Read the model definition and answer for the solid it produces. Units are mm, in the model's axes. Give positions to 0.01 mm unless a question says otherwise; leave off trailing zeros. Loops run counter-clockwise (first coordinate to the right, second up) from the corner with the lowest first, then second, coordinate; pieces in that order, holes last.
(1) Straight lines are drawn through the part: probe 1 along Z at (x, y) = (7.5, 479); probe 2 along X at (y, z) = (317.5, 20.05); probe 3 along X at (y, z) = (562, -23). For each, find the intervals that lie inside material, in ascending order.
(2) Find section B-B, the plane z = -14. Write down the section's boundary in (x, y).
(3) Find section A-A, the plane y = 378.5. Write down the section's boundary in (x, z).
(4) Each of these flat-tipped pins is pushed along its axis until it touches: P1, Ø4, axis at y = 452, z = -11, coming from the +X side; P2, Ø4, axis at x = 8, y = 305.5, coming from the -Z side; P3, Ø12, axis at x = -9, y = 530.5, coming from the -Z side. Where does it stop, or does it pass through?
```python
from build123d import *

# Parameters (mm, degrees)
F1_DEPTH = 609.6
F2_R     = 3.175
F3_DEPTH = 25.4
F4_R     = 2.54


with BuildPart() as f1:
    # F0 (on Front) → F1 (new body)
    with BuildSketch(Plane.XZ):
        with BuildLine():
            Line((-16.424578, 19.260229), (12.06593, 19.260229))
            Line((12.06593, 19.260229), (12.06593, 20.758829))
            Line((12.06593, 20.758829), (-16.653178, 20.758829))
            ThreePointArc((-16.653178, 20.758829), (-22.041332, 18.526982), (-24.273178, 13.138829))
            Line((-24.273178, 13.138829), (-24.273178, -23.307944))
            ThreePointArc((-24.273178, -23.307944), (-21.449279, -26.988121), (-17.163621, -25.212944))
            Line((-17.163621, -25.212944), (-4.463621, -3.215899))
            Line((-4.463621, -3.215899), (-5.761447, -2.466599))
            Line((-5.761447, -2.466599), (-18.034874, -23.724797))
            ThreePointArc((-18.034874, -23.724797), (-20.891979, -24.908249), (-22.774578, -22.454797))
            Line((-22.774578, -22.454797), (-22.774578, 12.910229))
            ThreePointArc((-22.774578, 12.910229), (-20.914706, 17.400357), (-16.424578, 19.260229))
        make_face()
    extrude(amount=-F1_DEPTH)

    # F2 (on face) → F3 (cut)
    with BuildSketch(Plane.XY.offset(20.758829)):
        with Locations((-0.63407, 12.7)):
            Circle(F2_R)
        with Locations((-0.63407, 38.1)):
            Circle(F2_R)
        with Locations((-0.63407, 63.5)):
            Circle(F2_R)
        with Locations((-0.63407, 88.9)):
            Circle(F2_R)
        with Locations((-0.63407, 114.3)):
            Circle(F2_R)
        with Locations((-0.63407, 139.7)):
            Circle(F2_R)
        with Locations((-0.63407, 165.1)):
            Circle(F2_R)
        with Locations((-0.63407, 190.5)):
            Circle(F2_R)
        with Locations((-0.63407, 215.9)):
            Circle(F2_R)
        with Locations((-0.63407, 241.3)):
            Circle(F2_R)
        with Locations((-0.63407, 266.7)):
            Circle(F2_R)
        with Locations((-0.63407, 292.1)):
            Circle(F2_R)
        with Locations((-0.63407, 317.5)):
            Circle(F2_R)
        with Locations((-0.63407, 342.9)):
            Circle(F2_R)
        with Locations((-0.63407, 368.3)):
            Circle(F2_R)
        with Locations((-0.63407, 393.7)):
            Circle(F2_R)
        with Locations((-0.63407, 419.1)):
            Circle(F2_R)
        with Locations((-0.63407, 444.5)):
            Circle(F2_R)
        with Locations((-0.63407, 469.9)):
            Circle(F2_R)
        with Locations((-0.63407, 495.3)):
            Circle(F2_R)
        with Locations((-0.63407, 520.7)):
            Circle(F2_R)
        with Locations((-0.63407, 546.1)):
            Circle(F2_R)
        with Locations((-0.63407, 571.5)):
            Circle(F2_R)
        with Locations((-0.63407, 596.9)):
            Circle(F2_R)
    extrude(amount=-F3_DEPTH, mode=Mode.SUBTRACT)

    # F4
    f4_edges = [f1.edges().sort_by_distance(p)[0] for p in [
        (12.06593, 0, 20.009529),
        (-5.112534, 0, -2.841249),
        (-5.112534, 609.6, -2.841249),
        (12.06593, 609.6, 20.009529),
    ]]
    fillet(f4_edges, radius=F4_R)


solid = f1.part
```
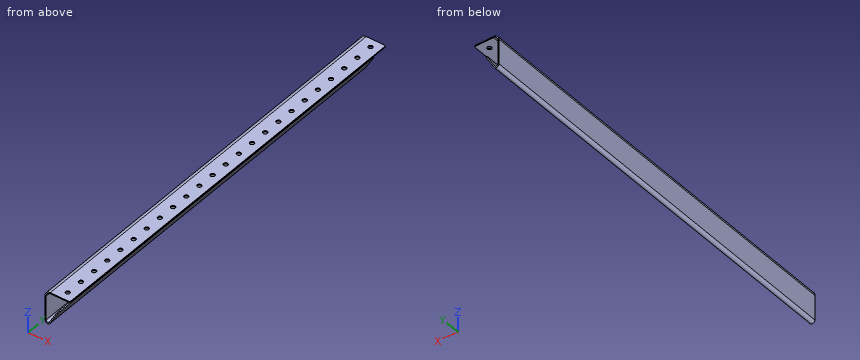
Entries:
1. probe 1: z = 19.26 to 20.76
1. probe 2: x = -19.86 to -3.81, 2.54 to 12.07
1. probe 3: x = -24.27 to -22.72, -17.62 to -15.89
2. outline: (-24.27, 0) - (-22.77, 0) - (-22.77, 609.6) - (-24.27, 609.6) - close; (-12.42, 0) - (-10.69, 0) - (-10.69, 609.6) - (-12.42, 609.6) - close
3. outline: (-24.27, -23.31) arc R3.81 ccw to (-17.16, -25.21) - (-4.46, -3.22) - (-5.76, -2.47) - (-18.03, -23.72) arc R2.54 cw to (-22.77, -22.45) - (-22.77, 12.91) arc R6.35 cw to (-16.42, 19.26) - (12.07, 19.26) - (12.07, 20.76) - (-16.65, 20.76) arc R7.62 ccw to (-24.27, 13.14) - close
4. P1: stops at x = -7.8
4. P2: stops at z = 19.26
4. P3: stops at z = -21.47
